Build history of the part. All positions in model axes, mm. Give positions to 0.01 mm unless a question says otherwise; leave off trailing zeros. Order: outer loops, then holes, each group sorted by start corner. A loop starts at its lowest first (then second) coordinate and runs counter-clockwise, first axis right, second up. Notation, with made-up numbers: (22, 32.25) - (75, 32.25) arc R16 cw to (75, 60.25) - close; hole circle Ø5 at (39, -10.5). An arc over 180 degrees is marked (long way). Answer in a Markdown table with one row per item.
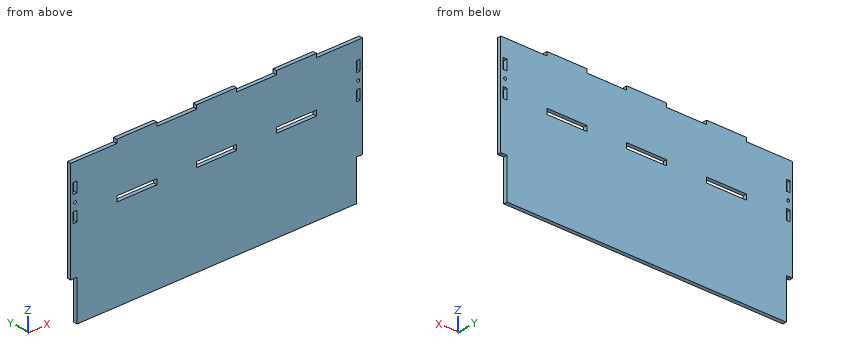
```python
from build123d import *

# Parameters (mm, degrees)
F0_R     = 1.8415
F0_W     = 51.054
F0_H     = 6.604
F0_W_2   = 50.8
F0_H_2   = 4.7625
F1_DEPTH = 4.7625


with BuildPart() as f1:
    # F0 (on Front) → F1 (new body)
    with BuildSketch(Plane.XZ):
        Polygon((-127, 88.9), (-182.5625, 88.9), (-182.5625, 66.802), (-177.673, 66.802), (-177.673, 53.848), (-182.5625, 53.848), (-182.5625, 35.052), (-177.673, 35.052), (-177.673, 22.098), (-182.5625, 22.098), (-182.5625, -37.973), (-177.673, -37.973), (-177.673, -88.9), (177.673, -88.9), (177.673, -37.973), (182.5625, -37.973), (182.5625, 22.098), (177.673, 22.098), (177.673, 35.052), (182.5625, 35.052), (182.5625, 53.848), (177.673, 53.848), (177.673, 66.802), (182.5625, 66.802), (182.5625, 88.9), (127, 88.9), (76.2, 88.9), (25.4, 88.9), (-25.4, 88.9), (-76.2, 88.9), align=None)
        with Locations((-180.18125, 44.45)):
            Circle(F0_R, mode=Mode.SUBTRACT)
        with Locations((-101.6, 28.575)):
            Rectangle(F0_W, F0_H, mode=Mode.SUBTRACT)
        with Locations((0, 28.575)):
            Rectangle(F0_W, F0_H, mode=Mode.SUBTRACT)
        with Locations((101.6, 28.575)):
            Rectangle(F0_W, F0_H, mode=Mode.SUBTRACT)
        with Locations((180.18125, 44.45)):
            Circle(F0_R, mode=Mode.SUBTRACT)
        with Locations((-101.6, 91.28125)):
            Rectangle(F0_W_2, F0_H_2)
        with Locations((0, 91.28125)):
            Rectangle(F0_W_2, F0_H_2)
        with Locations((101.6, 91.28125)):
            Rectangle(F0_W_2, F0_H_2)
        Polygon((-182.5625, 66.802), (-182.5625, 88.9), (-185.7375, 88.9), (-185.7375, -38.1), (-182.6895, -38.1), (-182.6895, -37.973), (-182.5625, -37.973), (-182.5625, 22.098), (-182.6895, 22.098), (-182.6895, 35.052), (-182.5625, 35.052), (-182.5625, 53.848), (-182.6895, 53.848), (-182.6895, 66.802), align=None)
        Polygon((185.7375, 88.9), (182.5625, 88.9), (182.5625, 66.802), (182.6895, 66.802), (182.6895, 53.848), (182.5625, 53.848), (182.5625, 35.052), (182.6895, 35.052), (182.6895, 22.098), (182.5625, 22.098), (182.5625, -37.973), (182.6895, -37.973), (182.6895, -38.1), (185.7375, -38.1), align=None)
    extrude(amount=F1_DEPTH)


solid = f1.part
```
1. Cut at C-C on z = -56. Write the cut outline in (x, y).
Check result:
| item | result |
|---|---|
| outline | (-177.67, -4.76) - (177.67, -4.76) - (177.67, 0) - (-177.67, 0) - close |
2. Cut at A-A on x = 10. Write the cut outline in (y, z).
Check result:
| item | result |
|---|---|
| outline | (-4.76, -88.9) - (0, -88.9) - (0, 25.27) - (-4.76, 25.27) - close; (-4.76, 31.88) - (0, 31.88) - (0, 93.66) - (-4.76, 93.66) - close |
3. Probe line 1 (Z direction, x = 126.5, y = -3.05); line 2 (Z direction, x = -151.5, y = -1.05); line 3 (X direction, y = -3.9, z = -70.5). List the from-to ranges inside material, lowest first.
Check result:
| item | result |
|---|---|
| line 1 | z = -88.9 to 25.27, 31.88 to 93.66 |
| line 2 | z = -88.9 to 88.9 |
| line 3 | x = -177.67 to 177.67 |
4. Drop flat-ended pins along their axis: P1, Ø2.5, axis at y = -3.5, z = 91, coming from the -X side; P2, Ø2, axis at y = -1.5, z = -49.5, coming from the -X side. Give the stop position or say it passes through.
Check result:
| item | result |
|---|---|
| P1 | stops at x = -127 |
| P2 | stops at x = -177.67 |
5. Cut at B-B on y = -2.2. Count the separate pieces of the cut face and the enclosed holes in it, and give its area (3 significant figures).
Check result:
| item | result |
|---|---|
| separate pieces | 1 |
| enclosed holes | 9 |
| area | 64,700 mm² |
